Geometry check sheet. Reference: the model listing, model coordinates, mm. Round coordinates to 2 decimals unless told otherwise and drop trailing zeros. Write each loop counter-clockwise with the first axis right and the second up, starting at its lowest first coordinate (ties: lowest second). Pieces come first, ordered by that corner, then holes. Notation, with made-up numbers: (33.5, 75.25) - (53.5, 75.25) arc R26 ccw to (53.5, 95.25) - close; hole circle Ø7 at (11, -7.5). An arc over 180 degrees is marked (long way). Return JSON: item names as keys, results as strings. Group by question number.
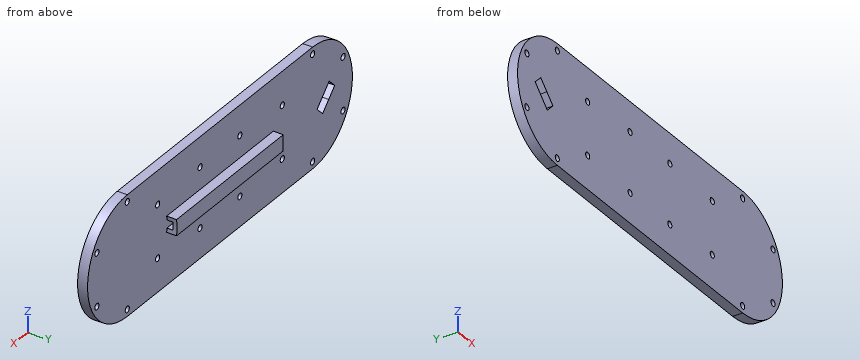
from build123d import *

# Parameters (mm, degrees)
SKETCH_1_R          = 1.55
EXTRUDE_2_DEPTH     = 5
SKETCH_2_R          = 1.55
CUT_EXTRUDE_2_DEPTH = 5
SKETCH_3_W          = 20
SKETCH_3_H          = 20
EXTRUDE_4_DEPTH     = 5
EXTRUDE_5_DEPTH     = 5
EXTRUDE_6_DEPTH     = 5
CUT_EXTRUDE_3_DEPTH = 150
SKETCH_8_W          = 8
SKETCH_8_H          = 5
CUT_EXTRUDE_4_DEPTH = 10
CUT_EXTRUDE_5_DEPTH = 10


with BuildPart() as part:
    # 草图1 → 凸台-拉伸2 (new body)
    with BuildSketch(Plane(origin=(0, 0, 0), x_dir=(1, 0, 0), z_dir=(0, 1, 0))):
        with BuildLine():
            Line((-70, 30), (70, 30))
            ThreePointArc((70, 30), (100, 0), (70, -30))
            Line((70, -30), (-70, -30))
            ThreePointArc((-70, -30), (-100, 0), (-70, 30))
        make_face()
        with Locations(Location((-15, 15, 0), (0, 0, 270))):
            Circle(SKETCH_1_R, mode=Mode.SUBTRACT)
        with Locations(Location((15, 15, 0), (0, 0, 270))):
            Circle(SKETCH_1_R, mode=Mode.SUBTRACT)
        with Locations(Location((15, -15, 0), (0, 0, 270))):
            Circle(SKETCH_1_R, mode=Mode.SUBTRACT)
        with Locations(Location((-15, -15, 0), (0, 0, 270))):
            Circle(SKETCH_1_R, mode=Mode.SUBTRACT)
        Polygon((-90, 0), (-90, 10), (-70, 10), (-70, -10), (-90, -10), align=None, mode=Mode.SUBTRACT)
        Polygon((90, 0), (90, 10), (70, 10), (70, -10), (90, -10), align=None, mode=Mode.SUBTRACT)
    extrude(amount=EXTRUDE_2_DEPTH)

    # 草图2 → 切除-拉伸2 (cut)
    with BuildSketch(Plane(origin=(0, 5, 0), x_dir=(1, 0, 0), z_dir=(0, 1, 0))):
        with Locations(Location((-70, 26.5, 0), (0, 0, 270))):
            Circle(SKETCH_2_R)
        with Locations(Location((-92.9496732, 13.25, 0), (0, 0, 270))):
            Circle(SKETCH_2_R)
        with Locations(Location((-92.9496732, -13.25, 0), (0, 0, 270))):
            Circle(SKETCH_2_R)
        with Locations(Location((-70, -26.5, 0), (0, 0, 270))):
            Circle(SKETCH_2_R)
        with Locations(Location((-47.0503268, -13.25, 0), (0, 0, 270))):
            Circle(SKETCH_2_R)
        with Locations(Location((-47.0503268, 13.25, 0), (0, 0, 270))):
            Circle(SKETCH_2_R)
        with Locations(Location((92.9496732, 13.25, 0), (0, 0, 270))):
            Circle(SKETCH_2_R)
        with Locations(Location((92.9496732, -13.25, 0), (0, 0, 270))):
            Circle(SKETCH_2_R)
        with Locations(Location((70, -26.5, 0), (0, 0, 270))):
            Circle(SKETCH_2_R)
        with Locations(Location((47.0503268, -13.25, 0), (0, 0, 270))):
            Circle(SKETCH_2_R)
        with Locations(Location((47.0503268, 13.25, 0), (0, 0, 270))):
            Circle(SKETCH_2_R)
        with Locations(Location((70, 26.5, 0), (0, 0, 270))):
            Circle(SKETCH_2_R)
    extrude(amount=-CUT_EXTRUDE_2_DEPTH, mode=Mode.SUBTRACT)

    # 草图3 → 凸台-拉伸4 (add)
    with BuildSketch(Plane(origin=(0, 5, 0), x_dir=(1, 0, 0), z_dir=(0, 1, 0))):
        with Locations((-80, 0)):
            Rectangle(SKETCH_3_W, SKETCH_3_H)
        with Locations((80, 0)):
            Rectangle(SKETCH_3_W, SKETCH_3_H)
    extrude(amount=-EXTRUDE_4_DEPTH)

    # 草图4 → 凸台-拉伸5 (add)
    with BuildSketch(Plane(origin=(0, 5, 0), x_dir=(1, 0, 0), z_dir=(0, 1, 0))):
        with BuildLine():
            Line((0, 4), (40.267862505, 4))
            ThreePointArc((40.267862505, 4), (40, 0), (40.267862505, -4))
            Line((40.267862505, -4), (0, -4))
            Line((0, -4), (-40.267862505, -4))
            ThreePointArc((-40.267862505, -4), (-40, 0), (-40.267862505, 4))
            Line((-40.267862505, 4), (0, 4))
        make_face()
    extrude(amount=EXTRUDE_5_DEPTH)

    # 草图6 → 凸台-拉伸6 (add)
    with BuildSketch(Plane(origin=(0, 5, 0), x_dir=(1, 0, 0), z_dir=(0, 1, 0))):
        Polygon((63.550267448, 4), (70, 4), (70, 0), (70, -4), (63.550267448, -4), align=None)
    extrude(amount=EXTRUDE_6_DEPTH)

    # 草图7 → 切除-拉伸3 (cut)
    with BuildSketch(Plane(origin=(70, 0, 0), x_dir=(0, 0, -1), z_dir=(1, 0, 0))):
        Polygon((2, 8), (0, 8), (-2, 8), (-2, 5), (0, 5), (2, 5), align=None)
    extrude(amount=-CUT_EXTRUDE_3_DEPTH, mode=Mode.SUBTRACT)

    # 草图8 → 切除-拉伸4 (cut)
    with BuildSketch(Plane(origin=(70, 0, 0), x_dir=(0, 0, -1), z_dir=(1, 0, 0))):
        with Locations((0, 7.5)):
            Rectangle(SKETCH_8_W, SKETCH_8_H)
    extrude(amount=-CUT_EXTRUDE_4_DEPTH, mode=Mode.SUBTRACT)

    # 草图9 → 切除-拉伸5 (cut)
    with BuildSketch(Plane.XZ):
        Polygon((-82.121320344, -2.121320344), (-86.717514421, 2.474873734), (-82.474873734, 6.717514421), (-77.878679656, 2.121320344), (-73.282485579, -2.474873734), (-77.525126266, -6.717514421), align=None)
    extrude(amount=-CUT_EXTRUDE_5_DEPTH, mode=Mode.SUBTRACT)


solid = part.part
1. Section check B-B (y = 3.5). State how many separate pieces and enclosed holes the cut face has, and give its area (3 significant figures).
2. Material ranges on line 1 along Z through (x, y) = (-70, 2.3); line 2 along Z through (x, y) = (23, 7.75); line 3 along X through (y, z) = (2, 13.25), recorded low to high.
3. Section check D-D (z = 19.5). Enter the section's corners in (x, y), and give its area (3 significant figures).
4. Section check A-A (x = -25.5). Enter the section's corners in (y, z), and give its area (3 significant figures).
5. Section check C-C (x = 52). Enter the section's corners in (y, z), and give its area (3 significant figures).
6. Depth check by flat-ended pin: pin 1 Ø1.5 at (x, y) = (2.5, 6) entering from +Z; pin 2 Ø12 at (x, z) = (-79, -22.5) entering from +Y; pin 3 Ø4 at (x, y) = (-14.5, 8.5) entering from -Z. Enter the tip coordinate at first touch or a pass-through.
Result sheet:
{
 "1": {"separate pieces": "1", "enclosed holes": "17", "area": "11,000 mm²"},
 "2": {"line 1": "z = -30 to -28.05, -24.95 to 24.95, 28.05 to 30", "line 2": "z = -4 to -2, 2 to 4", "line 3": "x = -96.92 to -94.5, -91.4 to -48.6, -45.5 to 45.5, 48.6 to 91.4, 94.5 to 96.92"},
 "3": {"outline": "(-92.8, 0) - (92.8, 0) - (92.8, 5) - (-92.8, 5) - close", "area": "928 mm²"},
 "4": {"outline": "(0, -30) - (5, -30) - (5, -4) - (10, -4) - (10, 4) - (5, 4) - (5, 30) - (0, 30) - close; hole (5, -2) - (8, -2) - (8, 2) - (5, 2) - close", "area": "328 mm²"},
 "5": {"outline": "(0, -30) - (5, -30) - (5, 30) - (0, 30) - close", "area": "300 mm²"},
 "6": {"pin 1": "stops at z = 4", "pin 2": "stops at y = 5", "pin 3": "stops at z = -4"}
}
